The drawing under review shows one solid part. Ordinate dimensions are in mm from its lowest x, y, z. A direction names the side the tool comes from. Round coordinates to 2 decimals unless told otherwise and drop trailing zeros. Order: outer loops, then holes, each group sorted by start corner. A loop starts at its lowest first (then second) coordinate and runs counter-clockwise, first axis right, second up. Notation, with made-up numbers: M 62.5,30 L 67.5,30 A16 ccw 67.5,48 Z; hole C -20.5,45.5 d10. An arc over 180 degrees is marked long. Answer as a JSON object with one key per item and string values. Group by question number.
1. Add section A-A on x = 3.5. State the section outline as (y, z) points (1 decimal).
2. Machinability: for the marked faces 1, 2, 3 and 4, which of the approach directions +Z, -Z, +X, -X, +Y, -Y give a long, thin tool a straight path to every point of the face, cutting with its end or side? Answer none if there is none.
3. Add section B-B on z = 5. State the section outline as (x, y) points (1 decimal).
4. To check wall thickness, follow probe 1 along X at (y, z) = (1.5, 2.5); probe 2 along Z at (x, y) = (5.5, 5.75); probe 3 along Y at (x, z) = (2, 2.75). State the ranges of each line that lie inside material, in increasing order. Write a range as [from, to].
5. Clearance check with flat-ended pins moving along their axes: P1, Ø1.6, axis at y = 3, z = 2.5, coming from the -X side; P2, Ø1, axis at y = 1.5, z = 2.5, coming from the +X side; P3, Ø0.6, axis at x = 5, z = 4.5, coming from the -Y side. State where each tip first meets the part, or that it passes through.
6. Add section C-C on z = 9. State the section outline as (x, y) points.
7. Add section D-D on x = 0.5. State the section outline as (y, z) points.
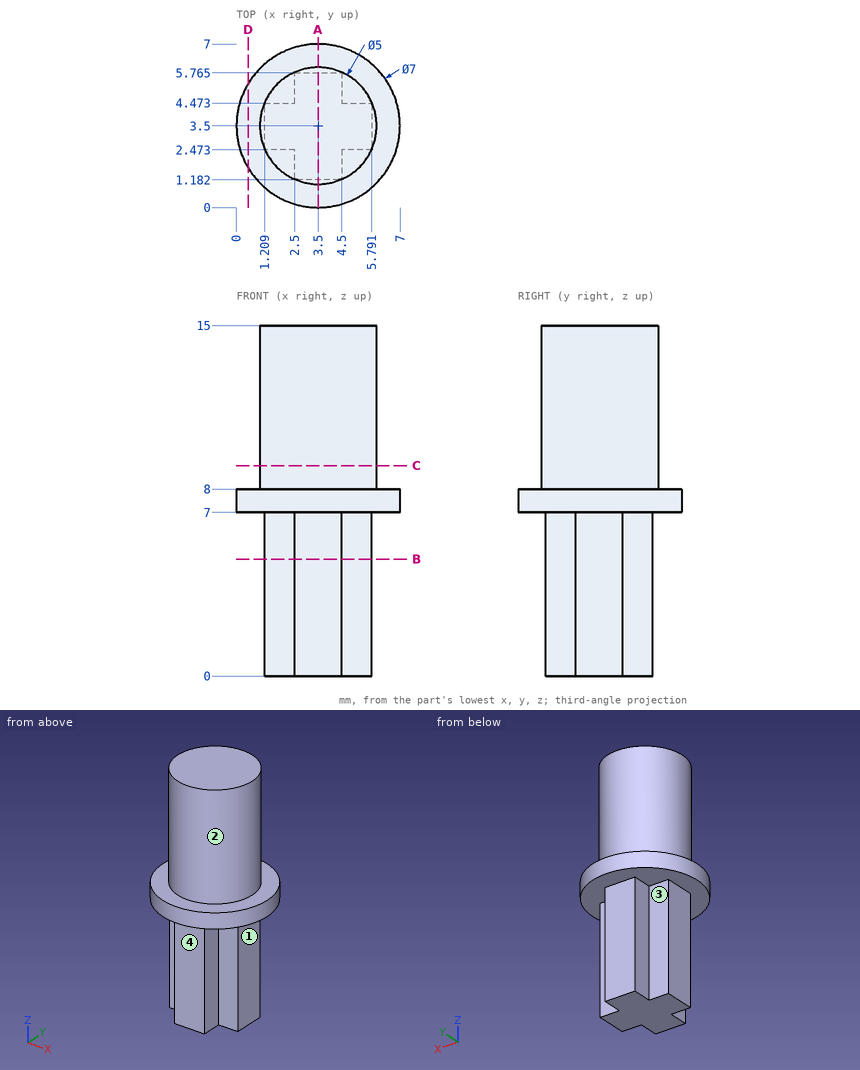
Recorded:
{
 "1": {"outline": "M 0,7 L 1.2,7 L 1.2,0 L 5.8,0 L 5.8,7 L 7,7 L 7,8 L 6,8 L 6,15 L 1,15 L 1,8 L 0,8 Z"},
 "2": {"face 1": "-Z, +X, +Y, -Y", "face 2": "+Z", "face 3": "-Z, -X, +Y", "face 4": "-Z, +X, -X, -Y"},
 "3": {"outline": "M 1.2,2.5 L 2.5,2.5 L 2.5,1.2 L 4.5,1.2 L 4.5,2.5 L 5.8,2.5 L 5.8,4.5 L 4.5,4.5 L 4.5,5.8 L 2.5,5.8 L 2.5,4.5 L 1.2,4.5 Z"},
 "4": {"probe 1": "x = [2.5, 4.5]", "probe 2": "z = [7, 8]", "probe 3": "y = [2.47, 4.47]"},
 "5": {"P1": "stops at x = 1.21", "P2": "stops at x = 4.5", "P3": "stops at y = 2.47"},
 "6": {"outline": "C 3.5,3.5 d5"},
 "7": {"outline": "M 1.7,7 L 5.3,7 L 5.3,8 L 1.7,8 Z"}
}
